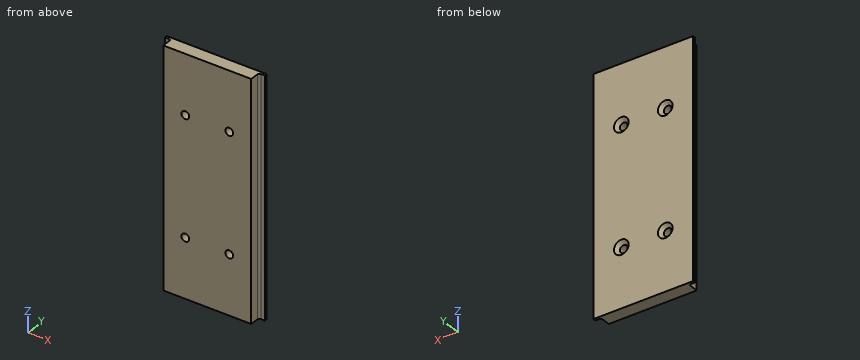
from build123d import *

# Parameters (mm, degrees)
BOSS_EXTRUDE1_DEPTH                               = 88.9
CSK_FOR_M2_5_FLAT_HEAD_MACHINE_SCREW1_D           = 2.9
CSK_FOR_M2_5_FLAT_HEAD_MACHINE_SCREW1_CSINK_D     = 5.5
CSK_FOR_M2_5_FLAT_HEAD_MACHINE_SCREW1_CSINK_ANGLE = 90


with BuildPart() as part:
    # Sketch1 → Boss-Extrude1 (new body)
    with BuildSketch(Plane.XY):
        with BuildLine():
            Line((-16.5, 3.25), (-16.5, 0))
            Line((-16.5, 0), (16.5, 0))
            Line((16.5, 0), (16.5, 3.25))
            ThreePointArc((16.5, 3.25), (16.719669914, 3.780330086), (17.25, 4))
            Line((17.25, 4), (18.75, 4))
            Line((18.75, 4), (18.75, 5))
            Line((18.75, 5), (-18.75, 5))
            Line((-18.75, 5), (-18.75, 4))
            Line((-18.75, 4), (-17.25, 4))
            ThreePointArc((-17.25, 4), (-16.719669914, 3.780330086), (-16.5, 3.25))
        make_face()
    extrude(amount=BOSS_EXTRUDE1_DEPTH)

    # CSK for M2.5 Flat Head Machine Screw1 (through all)
    with Locations(Plane(origin=(0, 5, 0), x_dir=(1, 0, 0), z_dir=(0, 1, 0))):
        with Locations((8.250631971, -22.223297508), (-8.250631971, -22.223297508), (-8.250631971, -66.676702492), (8.250631971, -66.676702492)):
            CounterSinkHole(CSK_FOR_M2_5_FLAT_HEAD_MACHINE_SCREW1_D / 2, CSK_FOR_M2_5_FLAT_HEAD_MACHINE_SCREW1_CSINK_D / 2, counter_sink_angle=CSK_FOR_M2_5_FLAT_HEAD_MACHINE_SCREW1_CSINK_ANGLE)


solid = part.part
Geometry check sheet. Reference: the model listing, model coordinates, mm. Give positions to 0.01 mm unless a question says otherwise; leave off trailing zeros. Order: outer loops, then holes, each group sorted by start corner. A loop starts at its lowest first (then second) coordinate and runs counter-clockwise, first axis right, second up.
1. Sectioned sample at A-A (y = 1). Record the boundary of the cut face in (x, z), then the cut area to 3 significant figures.
Completed:
outline: (-16.5, 0) - (16.5, 0) - (16.5, 88.9) - (-16.5, 88.9) - close; hole circle Ø2.9 at (-8.25, 22.22); hole circle Ø2.9 at (-8.25, 66.68); hole circle Ø2.9 at (8.25, 22.22); hole circle Ø2.9 at (8.25, 66.68)
area: 2,910 mm2
2. Scan lines: line 1 (X direction, y = 2.55, z = 22.5); line 2 (Z direction, x = 9, y = 1.3); line 3 (Z direction, x = 8.5, y = 2.1). Record each from-to range of solid material in increasing order.
Completed:
line 1: x = -16.5 to -9.67, -6.83 to 6.83, 9.67 to 16.5
line 2: z = 0 to 20.98, 23.46 to 65.44, 67.92 to 88.9
line 3: z = 0 to 20.79, 23.65 to 65.25, 68.11 to 88.9
3. Sectioned sample at B-B (z = 34.5). Record the boundary of the cut face in (x, y).
Completed:
outline: (-18.75, 4) - (-17.25, 4) arc R0.75 cw to (-16.5, 3.25) - (-16.5, 0) - (16.5, 0) - (16.5, 3.25) arc R0.75 cw to (17.25, 4) - (18.75, 4) - (18.75, 5) - (-18.75, 5) - close
4. Depth check by flat-ended pin: pin 1 (3.5 mm diameter, centred on x = -8.25, z = 66.68, fed in from +Y); pin 2 (0.8 mm diameter, centred on x = -18, z = 55, fed in from -Y); pin 3 (8 mm diameter, centred on x = -1.5, z = 48, fed in from -Y); pin 4 (2 mm diameter, centred on y = 1.5, z = 36.5, fed in from -X). Enter the tip coordinate at first touch or a pass-through.
Completed:
pin 1: stops at y = 4
pin 2: stops at y = 4
pin 3: stops at y = 0
pin 4: stops at x = -16.5
